Here's how the part is built. I have some questions about the finished solid (model axes, mm). Face numbers are marked on the shaded views. Coordinates: 2 decimals unless noted, no trailing zeros. Order: outer loops, then holes, each group sorted by start corner. A loop starts at its lowest first (then second) coordinate and runs counter-clockwise, first axis right, second up. Notation, with made-up numbers: (73, 76.25) -> (122, 76.25) arc R8 cw to (122, 91.25) -> close; hole circle Ø6 at (-8.75, 86.5). An arc over 180 degrees is marked (long way). One line per item, written item: value. Start each with the question number.
```python
from build123d import *

# Parameters (mm, degrees)
SKETCH1_R           = 0.5
BOSS_EXTRUDE1_DEPTH = 1.5875
FILLET1_R           = 6.35
FILLET2_R           = 0.127


with BuildPart() as part:
    # Sketch1 → Boss-Extrude1 (new body)
    with BuildSketch(Plane.XY):
        with BuildLine():
            Line((-1.190625, -6), (-1.190625, 5.90625))
            Line((-1.190625, 5.90625), (0, 10.66875))
            Line((0, 10.66875), (1.190625, 5.90625))
            Line((1.190625, 5.90625), (1.190625, -6))
            ThreePointArc((1.190625, -6), (0, -7.190625), (-1.190625, -6))
        make_face()
        with Locations((0, -6)):
            Circle(SKETCH1_R, mode=Mode.SUBTRACT)
    extrude(amount=-BOSS_EXTRUDE1_DEPTH)

    # Fillet1
    fillet1_edges = [part.edges().sort_by_distance(p)[0] for p in [
        (-1.190625, 5.90625, -0.79375),
        (1.190625, 5.90625, -0.79375),
    ]]
    fillet(fillet1_edges, radius=FILLET1_R)

    # Fillet2
    fillet2_edges = [part.edges().sort_by_distance(p)[0] for p in [
        (0, 10.66875, -0.79375),
    ]]
    fillet(fillet2_edges, radius=FILLET2_R)


solid = part.part
```
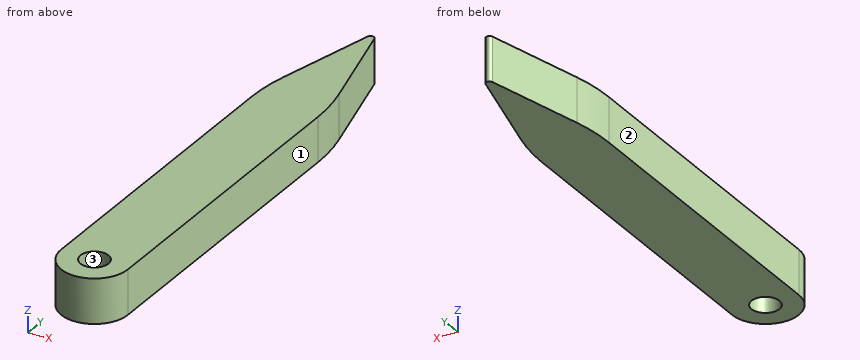
Q1. If we mould it in two halves opening along X, with no side actions, what happens to the marked faces 1, 2 and 3? For each: +X half, -X half, draft (parallel to the pull), parting line (faces both ways), or undercut.
Q2. Imagine slicing it at A-A (z = -0.6). Write out the boundary of the cut face in (x, y).
Q3. I need wall thicknesses on line 1 (Y direction, x = 0, z = -0.35); line 2 (X direction, y = 8, z = -0.7). Which ranges of each line are inside material? Lowest first, please.
Q4. Imagine slicing it at B-B (y = 8). Write out the boundary of the cut face in (x, z), plus the area to 3 significant figures.
Completed:
1. face 1: +X half
1. face 2: -X half
1. face 3: undercut
2. outline: (-1.19, -6) arc R1.19 ccw to (1.19, -6) -> (1.19, 5.12) arc R6.35 ccw to (1, 6.66) -> (0.12, 10.18) arc R0.13 ccw to (-0.12, 10.18) -> (-1, 6.66) arc R6.35 ccw to (-1.19, 5.12) -> close; hole circle Ø1 at (0, -6)
3. line 1: y = -7.19 to -6.5, -5.5 to 10.27
3. line 2: x = -0.67 to 0.67
4. outline: (-0.67, -1.59) -> (0.67, -1.59) -> (0.67, 0) -> (-0.67, 0) -> close
4. area: 2.12 mm2
